Autodesk Inventor part; units mm, degrees
ref_plane "YZ Plane" through (0, 0, 0) normal (1, 0, 0) x (0, 1, 0)
ref_plane "XZ Plane" through (0, 0, 0) normal (0, 1, 0) x (-1, 0, 0)
ref_plane "XY Plane" through (0, 0, 0) normal (0, 0, 1) x (1, 0, 0)
sketch "스케치1" plane through (0, 0, 0) normal (0, 1, 0) x (-1, 0, 0)
  line L0 (0, 0) -> (-54, 0)
  line L1 (-54, 0) -> (-54, -84)
  line L2 (-54, -84) -> (0, -84)
  line L3 (0, -84) -> (0, 0)
  line L4 (0, 0) -> (0, -2)
  line L5 (0, -2) -> (-2, -2)
  line L6 (-54, -84) -> (-54, -82)
  line L7 (-54, -82) -> (-52, -82)
  line L8 (-2, -2) -> (-52, -2)
  line L9 (-52, -2) -> (-52, -82)
  line L10 (-52, -82) -> (-2, -82)
  line L11 (-2, -82) -> (-2, -2)
  dimension "d0" = 54
  dimension "d1" = 84
  dimension "d2" = 2
  dimension "d3" = 2
  dimension "d4" = 2
  dimension "d5" = 2
extrude "돌출1" add sketch "스케치1" along normal blind 22 contours L3 L5 L8 L9 L7 L1 L0 | L3 L2 L1 L7 L10 L11 L5
extrude "돌출2" add sketch "스케치1" against normal blind 2
sketch "스케치2" plane through (0, 22, 0) normal (0, 0, 1) x (1, 0, 0)
  line L0 (0, -22) -> (7, -22)
  line L1 (0, -22) -> (7, -22) construction
  line L2 (7, -22) -> (8, -22)
  line L3 (8, -22) -> (8, -7)
  line L4 (8, -7) -> (18, -7)
  line L5 (18, -7) -> (18, -22)
  line L6 (18, -22) -> (8, -22)
  line L7 (8, -22) -> (18, -22)
  line L8 (18, -22) -> (18, -17)
  line L9 (18, -17) -> (8, -17)
  line L10 (8, -17) -> (8, -22)
  point P0 (8, -17)
  dimension "d10" = 7
  dimension "d11" = 0
  dimension "d12" = 1
  dimension "d13" = 15
  dimension "d14" = 10
  dimension "d15" = 5
extrude "돌출3" cut sketch "스케치2" against normal blind 2 contours L3 L4 L5 L9
properties part number "case"
Check sheet for the modelled part. Datum: model origin and axes. Units: mm. A direction names the side the tool comes from. Coordinates: 2 decimals unless noted, no trailing zeros. Write each loop counter-clockwise with the first axis right and the second up, starting at its lowest first coordinate (ties: lowest second). Pieces come first, ordered by that corner, then holes. Notation, with made-up numbers: M -13,-34 L -7,-34 A13 cw -7,-13 Z; hole C 57.5,41 d4. An arc over 180 degrees is marked long. Use one line per item in the form item = value.
Item 1: Release check for a two-part mould opening along X. For faces 4 (the face through (52, 11, -41)), 5 (the face through (54, 10, -41)), 6 (the face through (0, 10, -43)), 7 (the face through (27, 10, -84)) record: pulls with the +X half, pulls with the -X half, needs draft (parallel to the pull), parting line crosses it, or undercut.
Answer below:
face_4 = undercut
face_5 = pulls with the +X half
face_6 = pulls with the -X half
face_7 = needs draft
Item 2: Gauge pin test, flat end, axial feed: pin 1 Ø12 at (x, z) = (31, -52.5) entering from +Y. Record the tip position at first contact, or that the pin passes through.
Answer below:
pin_1 = 0
Item 3: Material ranges on L1, parallel to X at y = 19.75, z = -6.5; L2, parallel to Z at x = 4, y = 19.5; L3, parallel to Y at x = 25, z = -67, recorded low to high. Write a range as from..to.
Answer below:
L1 = 0..2, 52..54
L2 = -84..-82, -2..0
L3 = -2..0
Item 4: Sectioned sample at B-B, the plane y = 3.5. Record the cut outline in (x, z), and give its area (3 significant figures).
Answer below:
outline = M 0,-84 L 54,-84 L 54,0 L 0,0 Z; hole M 2,-82 L 52,-82 L 52,-2 L 2,-2 Z
area = 536 mm^2
Item 5: Sectioned sample at A-A, the plane y = 12.5. Record the cut outline in (x, z).
Answer below:
outline = M 0,-84 L 54,-84 L 54,0 L 18,0 L 18,-2 L 52,-2 L 52,-82 L 2,-82 L 2,-2 L 8,-2 L 8,0 L 0,0 Z
Item 6: Sectioned sample at C-C, the plane z = -73.5. Record the cut outline in (x, y).
Answer below:
outline = M 0,-2 L 54,-2 L 54,22 L 52,22 L 52,0 L 2,0 L 2,22 L 0,22 Z
Item 7: Sectioned sample at D-D, the plane x = 31. Record the cut outline in (y, z), and give its area (3 significant figures).
Answer below:
outline = M -2,-84 L 22,-84 L 22,-82 L 0,-82 L 0,-2 L 22,-2 L 22,0 L -2,0 Z
area = 256 mm^2
Item 8: Set-up check for faces 1 (the face through (27, 0, -41)), 2 (the face through (27, 10, 0)), 3 (the face through (8, 10, -1)): record each of +Z, -Z, +X, -X, +Y, -Y from which the full face is reachable in a straight line by a thin tool's end or side.
Answer below:
face_1 = +Y
face_2 = +Z, +X, -X, +Y, -Y
face_3 = +Z
